Verification items for the finished model (mm, model axes). Round coordinates to 2 decimals unless told otherwise and drop trailing zeros. Write each question's results on one line, items separated by ' | '.
```python
from build123d import *

# Parameters (mm, degrees)
SKETCH_1_W           = 360
SKETCH_1_H           = 40
EXTRUDE_1_DEPTH      = 3
SKETCH_2_W           = 16
SKETCH_2_H           = 27.5
EXTRUDE_2_DEPTH      = 3
SKETCH_3_R           = 1.5
SKETCH_3_R_2         = 4.5
SKETCH_3_R_3         = 3
CUT_EXTRUDE_1_DEPTH  = 4
SKETCH_6_W           = 0.5
SKETCH_6_H           = 12.5
CUT_EXTRUDE_4_DEPTH  = 10
CUT_EXTRUDE_10_DEPTH = 10
SKETCH_14_W          = 80
SKETCH_14_H          = 40
CUT_EXTRUDE_11_DEPTH = 10
SKETCH_15_R          = 2.05
CUT_EXTRUDE_12_DEPTH = 10
SKETCH_16_R          = 1.05
CUT_EXTRUDE_13_DEPTH = 10
SKETCH_17_W          = 20
SKETCH_17_H          = 2
EXTRUDE_3_DEPTH      = 3
SKETCH_18_W          = 20.1
SKETCH_18_H          = 2.1
CUT_EXTRUDE_14_DEPTH = 4
SKETCH_19_R          = 1
CUT_EXTRUDE_15_DEPTH = 3
CHAMFER_1_SIZE       = 10
CHAMFER_1_SIZE2      = 17.320508076
FILLET_2_R           = 2
SKETCH_22_R          = 1.55
CUT_EXTRUDE_17_DEPTH = 10
SKETCH_24_W          = 16.1
SKETCH_24_H          = 0.1
EXTRUDE_4_DEPTH      = 3
SKETCH_25_R          = 1
CUT_EXTRUDE_18_DEPTH = 10


with BuildPart() as part:
    # 草图1 → 凸台-拉伸1 (new body)
    with BuildSketch(Plane.XY):
        Rectangle(SKETCH_1_W, SKETCH_1_H)
    extrude(amount=EXTRUDE_1_DEPTH)

    # 草图2 → 凸台-拉伸2 (add)
    with BuildSketch(Plane.XY):
        with Locations((-188, -6.25)):
            Rectangle(SKETCH_2_W, SKETCH_2_H)
        with Locations((188, -6.25)):
            Rectangle(SKETCH_2_W, SKETCH_2_H)
    extrude(amount=EXTRUDE_2_DEPTH)

    # 草图3 → 切除-拉伸1 (cut, through all)
    with BuildSketch(Plane.XY.offset(3)):
        with Locations((-189, -12)):
            Circle(SKETCH_3_R)
        with Locations((-189, 4)):
            Circle(SKETCH_3_R)
        with Locations((-145, 0)):
            Circle(SKETCH_3_R_2)
        with Locations((189, 4)):
            Circle(SKETCH_3_R)
        with Locations((189, -12)):
            Circle(SKETCH_3_R)
        with Locations((72, 0)):
            Circle(SKETCH_3_R_3)
    extrude(amount=-CUT_EXTRUDE_1_DEPTH, mode=Mode.SUBTRACT)

    # 草图6 → 切除-拉伸4 (cut)
    with BuildSketch(Plane.XY.offset(3)):
        with Locations((-179.75, 13.75)):
            Rectangle(SKETCH_6_W, SKETCH_6_H)
        with Locations((179.75, 13.75)):
            Rectangle(SKETCH_6_W, SKETCH_6_H)
    extrude(amount=-CUT_EXTRUDE_4_DEPTH, mode=Mode.SUBTRACT)

    # 草图13 → 切除-拉伸10 (cut)
    with BuildSketch(Plane.XY.offset(3)):
        with BuildLine():
            Line((47, 3), (82, 3))
            ThreePointArc((82, 3), (85, 0), (82, -3))
            Line((82, -3), (47, -3))
            ThreePointArc((47, -3), (44, 0), (47, 3))
        make_face()
    extrude(amount=-CUT_EXTRUDE_10_DEPTH, mode=Mode.SUBTRACT)

    # 草图14 → 切除-拉伸11 (cut)
    with BuildSketch(Plane.XY.offset(3)):
        with Locations((-156, 0)):
            Rectangle(SKETCH_14_W, SKETCH_14_H)
    extrude(amount=-CUT_EXTRUDE_11_DEPTH, mode=Mode.SUBTRACT)

    # 草图15 → 切除-拉伸12 (cut)
    with BuildSketch(Plane.XY.offset(3)):
        with Locations((-85, 0)):
            Circle(SKETCH_15_R)
        with Locations((54, 0)):
            Circle(SKETCH_15_R)
        with Locations((-15.5, 0)):
            Circle(SKETCH_15_R)
    extrude(amount=-CUT_EXTRUDE_12_DEPTH, mode=Mode.SUBTRACT)

    # 草图16 → 切除-拉伸13 (cut)
    with BuildSketch(Plane(origin=(0, 0, 0), x_dir=(-1, 0, 0), z_dir=(0, 0, -1))):
        with Locations((-66.215, -17.5)):
            Circle(SKETCH_16_R)
        with Locations((-46.215, -17.5)):
            Circle(SKETCH_16_R)
        with Locations((-26.215, -17.5)):
            Circle(SKETCH_16_R)
        with Locations((-6.215, -17.5)):
            Circle(SKETCH_16_R)
        with Locations((13.785, -17.5)):
            Circle(SKETCH_16_R)
        with Locations((33.785, -17.5)):
            Circle(SKETCH_16_R)
        with Locations((53.785, -17.5)):
            Circle(SKETCH_16_R)
    extrude(amount=-CUT_EXTRUDE_13_DEPTH, mode=Mode.SUBTRACT)

    # 草图17 → 凸台-拉伸3 (add)
    with BuildSketch(Plane(origin=(0, 0, 0), x_dir=(-1, 0, 0), z_dir=(0, 0, -1))):
        with Locations((-55.215, 21)):
            Rectangle(SKETCH_17_W, SKETCH_17_H)
        with Locations((-21.215, 21)):
            Rectangle(SKETCH_17_W, SKETCH_17_H)
        with Locations((12.785, 21)):
            Rectangle(SKETCH_17_W, SKETCH_17_H)
        with Locations((46.785, 21)):
            Rectangle(SKETCH_17_W, SKETCH_17_H)
    extrude(amount=-EXTRUDE_3_DEPTH)

    # 草图18 → 切除-拉伸14 (cut, through all)
    with BuildSketch(Plane(origin=(0, 0, 0), x_dir=(-1, 0, 0), z_dir=(0, 0, -1))):
        with Locations((37.785, -14)):
            Rectangle(SKETCH_18_W, SKETCH_18_H)
        with Locations((-50.215, -14)):
            Rectangle(SKETCH_18_W, SKETCH_18_H)
        with Locations((-6.215, -14)):
            Rectangle(SKETCH_18_W, SKETCH_18_H)
    extrude(amount=-CUT_EXTRUDE_14_DEPTH, mode=Mode.SUBTRACT)

    # 草图19 → 切除-拉伸15 (cut)
    with BuildSketch(Plane(origin=(0, 0, 0), x_dir=(-1, 0, 0), z_dir=(0, 0, -1))):
        with Locations((-59.265, -12.95)):
            Circle(SKETCH_19_R)
        with Locations((-59.265, -15.05)):
            Circle(SKETCH_19_R)
        with Locations((-41.165, -12.95)):
            Circle(SKETCH_19_R)
        with Locations((-41.165, -15.05)):
            Circle(SKETCH_19_R)
        with Locations((-15.265, -12.95)):
            Circle(SKETCH_19_R)
        with Locations((-15.265, -15.05)):
            Circle(SKETCH_19_R)
        with Locations((2.835, -12.95)):
            Circle(SKETCH_19_R)
        with Locations((2.835, -15.05)):
            Circle(SKETCH_19_R)
        with Locations((28.735, -12.95)):
            Circle(SKETCH_19_R)
        with Locations((28.735, -15.05)):
            Circle(SKETCH_19_R)
        with Locations((46.835, -12.95)):
            Circle(SKETCH_19_R)
        with Locations((46.835, -15.05)):
            Circle(SKETCH_19_R)
    extrude(amount=-CUT_EXTRUDE_15_DEPTH, mode=Mode.SUBTRACT)

    # 倒角1
    chamfer_1_edges = [part.edges().sort_by_distance(p)[0] for p in [
        (179.5, 20, 1.5),
    ]]
    chamfer_1_side = [part.faces().sort_by_distance(p)[0] for p in [
        (179.5, 13.75, 1.5),
    ]]
    chamfer(chamfer_1_edges, length=CHAMFER_1_SIZE, length2=CHAMFER_1_SIZE2, reference=chamfer_1_side[0])

    # 圆角2
    fillet_2_edges = [part.edges().sort_by_distance(p)[0] for p in [
        (-116, 20, 1.5),
        (-116, -20, 1.5),
        (196, -20, 1.5),
        (196, 7.5, 1.5),
        (179.5, 10, 1.5),
        (162.179491924, 20, 1.5),
    ]]
    fillet(fillet_2_edges, radius=FILLET_2_R)

    # 草图22 → 切除-拉伸17 (cut)
    with BuildSketch(Plane(origin=(0, 0, 0), x_dir=(-1, 0, 0), z_dir=(0, 0, -1))):
        with Locations((79, 8)):
            Circle(SKETCH_22_R)
        with Locations((79, -8)):
            Circle(SKETCH_22_R)
    extrude(amount=-CUT_EXTRUDE_17_DEPTH, mode=Mode.SUBTRACT)

    # 草图24 → 凸台-拉伸4 (add)
    with BuildSketch(Plane(origin=(0, 0, 0), x_dir=(-1, 0, 0), z_dir=(0, 0, -1))):
        with Locations((-50.215, -13)):
            Rectangle(SKETCH_24_W, SKETCH_24_H)
        with Locations((-50.215, -15)):
            Rectangle(SKETCH_24_W, SKETCH_24_H)
        with Locations((-6.215, -13)):
            Rectangle(SKETCH_24_W, SKETCH_24_H)
        with Locations((-6.215, -15)):
            Rectangle(SKETCH_24_W, SKETCH_24_H)
        with Locations((37.785, -13)):
            Rectangle(SKETCH_24_W, SKETCH_24_H)
        with Locations((37.785, -15)):
            Rectangle(SKETCH_24_W, SKETCH_24_H)
    extrude(amount=-EXTRUDE_4_DEPTH)

    # 草图25 → 切除-拉伸18 (cut)
    with BuildSketch(Plane(origin=(0, 0, 0), x_dir=(-1, 0, 0), z_dir=(0, 0, -1))):
        with Locations((-65.215, 20)):
            Circle(SKETCH_25_R)
        with Locations((-45.215, 20)):
            Circle(SKETCH_25_R)
        with Locations((-31.215, 20)):
            Circle(SKETCH_25_R)
        with Locations((-11.215, 20)):
            Circle(SKETCH_25_R)
        with Locations((2.785, 20)):
            Circle(SKETCH_25_R)
        with Locations((22.785, 20)):
            Circle(SKETCH_25_R)
        with Locations((36.785, 20)):
            Circle(SKETCH_25_R)
        with Locations((56.785, 20)):
            Circle(SKETCH_25_R)
    extrude(amount=-CUT_EXTRUDE_18_DEPTH, mode=Mode.SUBTRACT)


solid = part.part
```
(1) Go/stop test with flat-tipped pins: pin 1 Ø1.1 at (y, z) = (21.5, 1.5) entering from -X (3 decimals); pin 2 Ø1.9 at (x, y) = (-53.785, -17.5) entering from +Z; pin 3 Ø1.1 at (y, z) = (21.5, 1.5) entering from +X (3 decimals); pin 4 Ø1.5 at (x, z) = (69, 2) entering from +Y. Record where each tip stops, or that it passes through.
Answer:
pin 1: x = -56.785 | pin 2: through | pin 3: x = 65.215 | pin 4: y = 20
(2) Section check A-A (z = 2.15). State how many separate pieces and enclosed holes the cut face has, plus the area to 3 significant figures.
Answer:
separate pieces: 1 | enclosed holes: 17 | area: 11,900 mm2
(3) Thickness scan on L1, parallel to Y at x = 49, z = 0.5; L2, parallel to Y at x = 189, z = 0.6; L3, parallel to Y at x = -85, z = 1.15. Record the ranges inside material, lowest first.
Answer:
L1: -20 to -14.95, -13.05 to -3, 3 to 22 | L2: -20 to -13.5, -10.5 to 2.5, 5.5 to 7.5 | L3: -20 to -2.05, 2.05 to 20
